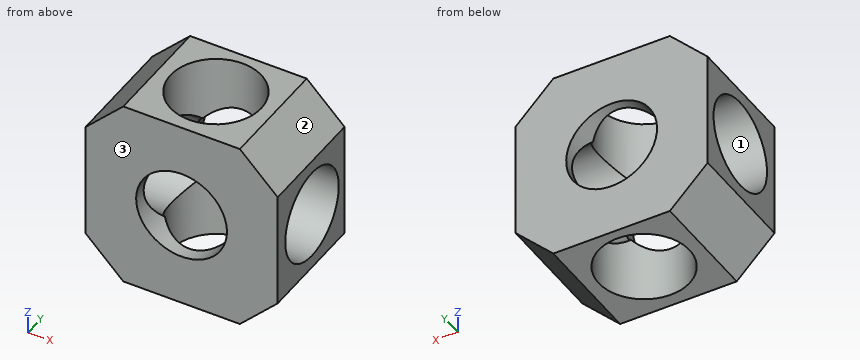
from build123d import *

# Parameters (mm, degrees)
SKETCH1_W           = 8.466666666
SKETCH1_H           = 8.466666667
BOSS_EXTRUDE1_DEPTH = 5
CHAMFER1_SIZE       = 1.666666667
SKETCH2_R           = 2
CUT_EXTRUDE1_DEPTH  = 10
SKETCH3_R           = 2
CUT_EXTRUDE2_DEPTH  = 12.317961286
SKETCH4_R           = 2
CUT_EXTRUDE3_DEPTH  = 10


with BuildPart() as part:
    # Sketch1 → Boss-Extrude1 (new body)
    with BuildSketch(Plane(origin=(0, 0, 0), x_dir=(1, 0, 0), z_dir=(0, 1, 0))):
        with Locations((-1.371290047, 0.771071428)):
            Rectangle(SKETCH1_W, SKETCH1_H)
    extrude(amount=BOSS_EXTRUDE1_DEPTH)

    # Chamfer1
    chamfer1_edges = [part.edges().sort_by_distance(p)[0] for p in [
        (2.862043286, 2.5, 3.462261905),
        (-5.60462338, 2.5, 3.462261905),
        (-5.60462338, 2.5, -5.004404762),
        (2.862043286, 2.5, -5.004404762),
    ]]
    chamfer(chamfer1_edges, length=CHAMFER1_SIZE)

    # Sketch2 → Cut-Extrude1 (cut)
    with BuildSketch(Plane(origin=(2.862043286, 0, 0), x_dir=(0, 0, -1), z_dir=(1, 0, 0))):
        with Locations((0.772738095, 2.565)):
            Circle(SKETCH2_R)
    extrude(amount=-CUT_EXTRUDE1_DEPTH, mode=Mode.SUBTRACT)

    # Sketch3 → Cut-Extrude2 (cut, through all)
    with BuildSketch(Plane.XY.offset(3.462261905)):
        with Locations((-1.36962338, 2.565)):
            Circle(SKETCH3_R)
    extrude(amount=-CUT_EXTRUDE2_DEPTH, mode=Mode.SUBTRACT)

    # Sketch4 → Cut-Extrude3 (cut)
    with BuildSketch(Plane(origin=(0, 5, 0), x_dir=(1, 0, 0), z_dir=(0, 1, 0))):
        with Locations(Location((-1.372956714, 0.772738095, 0), (0, 0, 270))):
            Circle(SKETCH4_R)
    extrude(amount=-CUT_EXTRUDE3_DEPTH, mode=Mode.SUBTRACT)


solid = part.part
Input: part model. Units: mm. Frame: model coordinates. Face numbers are marked on the shaded views. Give positions to 0.01 mm unless a question says otherwise; leave off trailing zeros. Order: outer loops, then holes, each group sorted by start corner. A loop starts at its lowest first (then second) coordinate and runs counter-clockwise, first axis right, second up. Notation, with made-up numbers: M 17.25,-9 L 73.25,-9 A29 ccw 73.25,11 Z; hole C 18.25,50.25 d3. An arc over 180 degrees is marked long. Answer as a JSON object with one key per item and string values.
1. Cut plane A-A, the plane y = 3.25. Output: boundary loops of the cut face in (x, z).
Result sheet:
{"outline": "M -5.6,-3.34 L -3.94,-5 L -3.25,-5 L -3.25,-2.65 L -5.6,-2.65 Z; M -5.6,1.11 L -3.25,1.11 L -3.25,3.46 L -3.94,3.46 L -5.6,1.8 Z; M 0.51,-5 L 1.2,-5 L 2.86,-3.34 L 2.86,-2.65 L 0.51,-2.65 Z; M 0.51,1.11 L 2.86,1.11 L 2.86,1.8 L 1.2,3.46 L 0.51,3.46 Z"}
2. Ray query, line 1 (Z direction, x = -5, y = 3.8); line 2 (Y direction, x = 0, z = 1.75); line 3 (X direction, y = 3.85, z = -3.75). Return the intervals inside material, ascending. Write a range as [from, to].
Result sheet:
{"line 1": "[-3.94, -2.35], [0.8, 2.4]", "line 2": "[0, 1.11], [4.02, 5]", "line 3": "[-5.19, -2.9], [0.16, 2.45]"}
3. Cut plane B-B, the plane x = -2. Output: boundary loops of the cut face in (y, z), and give its area (3 significant figures).
Result sheet:
{"outline": "M 0,-5 L 0.67,-5 L 0.67,-2.67 L 0,-2.67 Z; M 0,1.13 L 0.67,1.13 L 0.67,3.46 L 0,3.46 Z; M 4.46,-5 L 5,-5 L 5,-2.67 L 4.46,-2.67 Z; M 4.46,1.13 L 5,1.13 L 5,3.46 L 4.46,3.46 Z", "area": "5.62 mm²"}
4. Cut plane D-D, the plane x = 2.25. Output: boundary loops of the cut face in (y, z) (3 decimals), and give its area (3 significant figures).
Result sheet:
{"outline": "M 0,-3.95 L 5,-3.95 L 5,2.408 L 0,2.408 Z; hole C 2.565,-0.773 d4", "area": "19.2 mm²"}
5. Pull-direction query (Y, two-part tool) for the marked faces 1, 2 and 3; classes: +Y half, -Y half, draft (parallel to the pull), parting line (faces both ways), or undercut.
Result sheet:
{"face 1": "undercut", "face 2": "draft", "face 3": "-Y half"}
6. Cut plane C-C, the plane z = -1.25. Output: boundary loops of the cut face in (x, y).
Result sheet:
{"outline": "M -5.6,0 L -3.32,0 L -3.32,0.62 L -5.6,0.62 Z; M -5.6,4.51 L -3.32,4.51 L -3.32,5 L -5.6,5 Z; M 0.57,0 L 2.86,0 L 2.86,0.62 L 0.57,0.62 Z; M 0.57,4.51 L 2.86,4.51 L 2.86,5 L 0.57,5 Z"}
7. First-contact query: P1, Ø3, axis at x = -1.37, y = 2.56, coming from the -Z side. Flat tip, straight axial feed; report the tip coordinate or a pass-through.
Result sheet:
{"P1": "through"}
